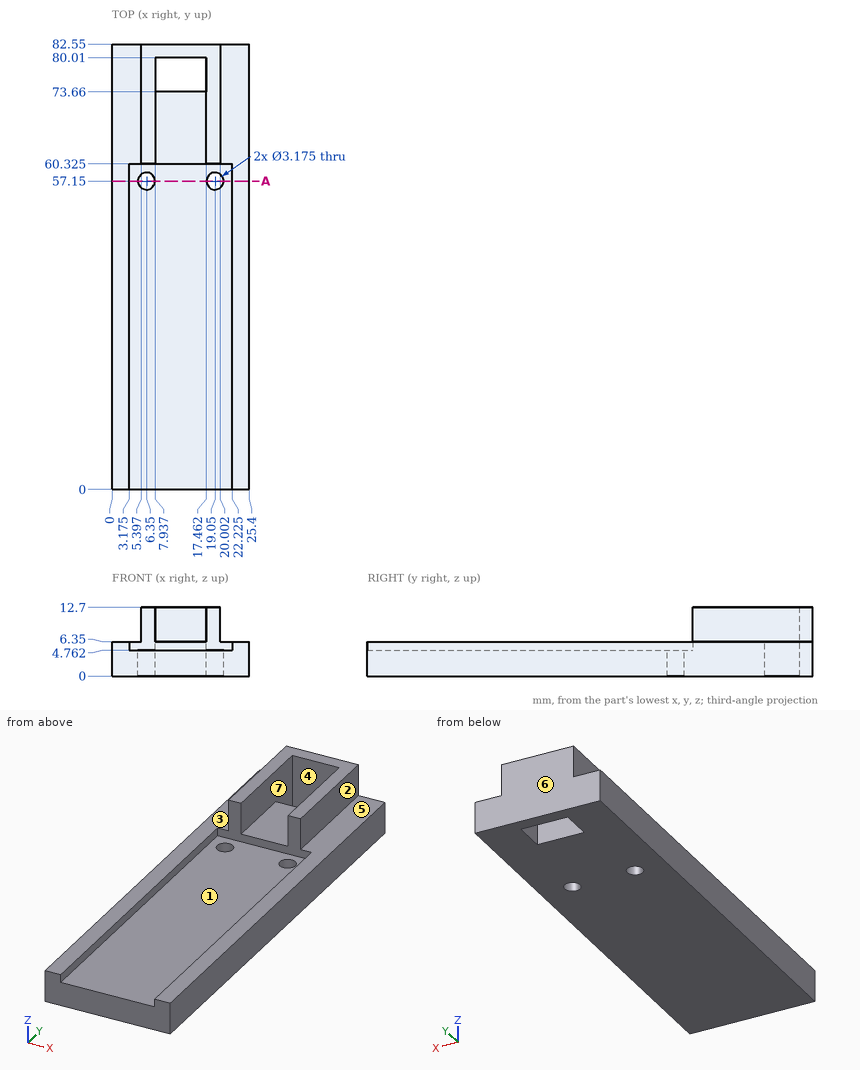
Part print with two shaded views. Sizes in mm from the minimum x, y, z corner. A direction names the side the tool comes from. Round coordinates to 2 decimals unless told otherwise and drop trailing zeros.
Item 1: Saw through at A-A (y = 57.15). State how many separate pieces and enclosed holes the cut face has, then the cut area to 3 significant figures.
Item 2: Two-plate mould, pull along Y, no slides. Class the marked faces 4, 5, 6 and 7: released by +Y, released by -Y, zero draft, split by the parting line, or undercut.
Item 3: Which spindle directions (+Z, -Z, +X, -X, +Y, -Y) get a long thin tool onto all of the face, cutting with end or side? Do the marked faces 1, 2 and 3. Say none if no direction does.
Item 4: Drill centre lines: line 1 along X through (y, z) = (73, 7.5); line 2 along X through (y, z) = (74, 1); line 3 along Y through (x, z) = (19.05, 2.6). Where is each one in solid material? Low to high.
Item 5: Pin check, flat tips, straight feed: P1, Ø4, axis at x = 6.35, y = 57.15, coming from the +Z side; P2, Ø3, axis at x = 12, y = 65, coming from the +Z side; P3, Ø4.5, axis at x = 24, y = 46, coming from the +Z side. Stop position of each tip, or through.
Worked answers:
1. separate pieces: 3
1. enclosed holes: 0
1. area: 101 mm2
2. face 4: undercut
2. face 5: zero draft
2. face 6: released by +Y
2. face 7: undercut
3. face 1: +Z, -Y
3. face 2: +Z, +X, +Y, -Y
3. face 3: +Z, -X, +Y, -Y
4. line 1: x = 5.4 to 7.94, 17.46 to 20
4. line 2: x = 0 to 7.94, 17.46 to 25.4
4. line 3: y = 0 to 55.56, 58.74 to 82.55
5. P1: stops at z = 4.76
5. P2: stops at z = 6.35
5. P3: stops at z = 6.35
